Verification items for the finished model (mm, model axes). A direction names the side the tool comes from. Round coordinates to 2 decimals unless told otherwise and drop trailing zeros. Write each loop counter-clockwise with the first axis right and the second up, starting at its lowest first coordinate (ties: lowest second). Pieces come first, ordered by that corner, then holes. Notation, with made-up numbers: M 66.25,51.25 L 73.25,51.25 A25 ccw 73.25,71.25 Z; hole C 5.25,48.5 d10. An arc over 180 degrees is marked long. Answer in a Markdown table with one row per item. Add a question column.
1. Material ranges on probe 1 along Z at (x, y) = (9.5, 5); probe 2 along Y at (x, z) = (-11, 78); probe 3 along Z at (x, y) = (-2, -17.5), recorded low to high.
2. Draft check along Y on faces 1 (the flat face through (0, -13, 70)), 2 (the cylindrical face through (-11.54, 16.61, 75.07)), 3 (the cylindrical face through (15.24, -6.32, 87.4)), 4 (the cylindrical face through (-6.466, -2.681, 12.325)). Enter one of: pulls with the +Y half, pulls with the -Y half, needs draft (parallel to the pull), parting line crosses it, or undercut.
3. Go/stop test with flat-tipped pins: pin 1 Ø4.5 at (x, y) = (11, -19.05) entering from +Z; pin 2 Ø7 at (x, y) = (3.5, -1.5) entering from -Z; pin 3 Ø6 at (x, y) = (-11, 19.05) entering from -Z; pin 4 Ø1.5 at (y, z) = (-4, 52.5) entering from +X. Record where each tip stops, or that it passes through.
4. Set-up check for faces 5 (the cylindrical face through (19.5, 0.1, 75.1)), 6 (the flat face through (-6.4, 3.3, 0)), 7 (the flat face through (13, -13, 80)), 8 (the cylindrical face through (12.932, -5.362, 14.79)), 9 (the cylindrical face through (-2.17, -9.76, 49.72)): record each of +Z, -Z, +X, -X, +Y, -Y from which the full face is reachable in a straight line by a thin tool's end or side.
5. Sectioned sample at A-A on y = 0. Record the cut outline in (x, z), plus the area to 4 significant figures.
6. Sectioned sample at B-B on x = 22. Record the cut outline in (y, z), plus the area to 3 significant figures.
7. Sectioned sample at D-D on x = 0. Record the cut outline in (y, z).
8. Sectioned sample at C-C on z = 15. Record the cut outline in (x, y), plus the area to 3 significant figures.
```python
from build123d import *

# Parameters (mm, degrees)
SCHIZZO1_R                   = 14
ESTRUSIONE_ESTRUSIONE1_DEPTH = 30
SCHIZZO2_R                   = 10
ESTRUSIONE_ESTRUSIONE2_DEPTH = 40
SCHIZZO3_R                   = 30
ESTRUSIONE_ESTRUSIONE3_DEPTH = 10
SCHIZZO4_R                   = 16.5
ESTRUSIONE_ESTRUSIONE4_DEPTH = 15
SCHIZZO5_R                   = 7
TAGLIO_ESTRUSIONE1_DEPTH     = 25
SCHIZZO6_R                   = 2.5
TAGLIO_ESTRUSIONE2_DEPTH     = 10


with BuildPart() as part:
    # Schizzo1 → Estrusione-Estrusione1 (new body)
    with BuildSketch(Plane.XY):
        Circle(SCHIZZO1_R)
    extrude(amount=ESTRUSIONE_ESTRUSIONE1_DEPTH)

    # Schizzo2 → Estrusione-Estrusione2 (add)
    with BuildSketch(Plane.XY.offset(30)):
        Circle(SCHIZZO2_R)
    extrude(amount=ESTRUSIONE_ESTRUSIONE2_DEPTH)

    # Schizzo3 → Estrusione-Estrusione3 (add)
    with BuildSketch(Plane.XY.offset(70)):
        Circle(SCHIZZO3_R)
    extrude(amount=ESTRUSIONE_ESTRUSIONE3_DEPTH)

    # Schizzo4 → Estrusione-Estrusione4 (add)
    with BuildSketch(Plane.XY.offset(80)):
        Circle(SCHIZZO4_R)
    extrude(amount=ESTRUSIONE_ESTRUSIONE4_DEPTH)

    # Schizzo5 → Taglio-Estrusione1 (cut)
    with BuildSketch(Plane(origin=(0, 0, 0), x_dir=(-1, 0, 0), z_dir=(0, 0, -1))):
        Circle(SCHIZZO5_R)
    extrude(amount=-TAGLIO_ESTRUSIONE1_DEPTH, mode=Mode.SUBTRACT)

    # Schizzo6 → Taglio-Estrusione2 (cut)
    with BuildSketch(Plane.XY.offset(80)):
        with Locations((22, 0)):
            Circle(SCHIZZO6_R)
        with Locations((11, 19.052558883)):
            Circle(SCHIZZO6_R)
        with Locations((-11, 19.052558883)):
            Circle(SCHIZZO6_R)
        with Locations((-22, 0)):
            Circle(SCHIZZO6_R)
        with Locations((-11, -19.052558883)):
            Circle(SCHIZZO6_R)
        with Locations((11, -19.052558883)):
            Circle(SCHIZZO6_R)
    extrude(amount=-TAGLIO_ESTRUSIONE2_DEPTH, mode=Mode.SUBTRACT)


solid = part.part
```
Geometry check:
| question | item | result |
|---|---|---|
| 1 | probe 1 | z = 0 to 30, 70 to 95 |
| 1 | probe 2 | y = -27.91 to -21.55, -16.55 to 16.55, 21.55 to 27.91 |
| 1 | probe 3 | z = 70 to 80 |
| 2 | face 1 | needs draft |
| 2 | face 2 | undercut |
| 2 | face 3 | parting line crosses it |
| 2 | face 4 | undercut |
| 3 | pin 1 | passes through |
| 3 | pin 2 | stops at z = 0 |
| 3 | pin 3 | stops at z = 70 |
| 3 | pin 4 | stops at x = 9.46 |
| 4 | face 5 | +Z, -Z |
| 4 | face 6 | -Z, +X, -X, +Y, -Y |
| 4 | face 7 | +Z |
| 4 | face 8 | -Z |
| 4 | face 9 | none |
| 5 | outline | M -30,70 L -24.5,70 L -24.5,80 L -30,80 Z; M -19.5,70 L -10,70 L -10,30 L -14,30 L -14,0 L -7,0 L -7,25 L 7,25 L 7,0 L 14,0 L 14,30 L 10,30 L 10,70 L 19.5,70 L 19.5,80 L 16.5,80 L 16.5,95 L -16.5,95 L -16.5,80 L -19.5,80 Z; M 24.5,70 L 30,70 L 30,80 L 24.5,80 Z |
| 5 | area | 2,285 mm2 |
| 6 | outline | M -20.4,70 L -2.5,70 L -2.5,80 L -20.4,80 Z; M 2.5,70 L 20.4,70 L 20.4,80 L 2.5,80 Z |
| 6 | area | 358 mm2 |
| 7 | outline | M -30,70 L -10,70 L -10,30 L -14,30 L -14,0 L -7,0 L -7,25 L 7,25 L 7,0 L 14,0 L 14,30 L 10,30 L 10,70 L 30,70 L 30,80 L 16.5,80 L 16.5,95 L -16.5,95 L -16.5,80 L -30,80 Z |
| 8 | outline | C 0,0 d28; hole C 0,0 d14 |
| 8 | area | 462 mm2 |
